Study the drawing (mm; zero at the part's minimum x, y, z) and answer. A direction names the side the tool comes from. Coordinates: 2 decimals unless noted, no trailing zeros. Order: outer loops, then holes, each group sorted by start corner. A loop starts at its lowest first (then second) coordinate and runs counter-clockwise, first axis right, second up. Notation, with made-up numbers: M 62,76 L 107,76 A17 ccw 107,81 Z; hole C -15,64.5 d2. An arc over 180 degrees is marked long. Put each result on its own line as item: value.
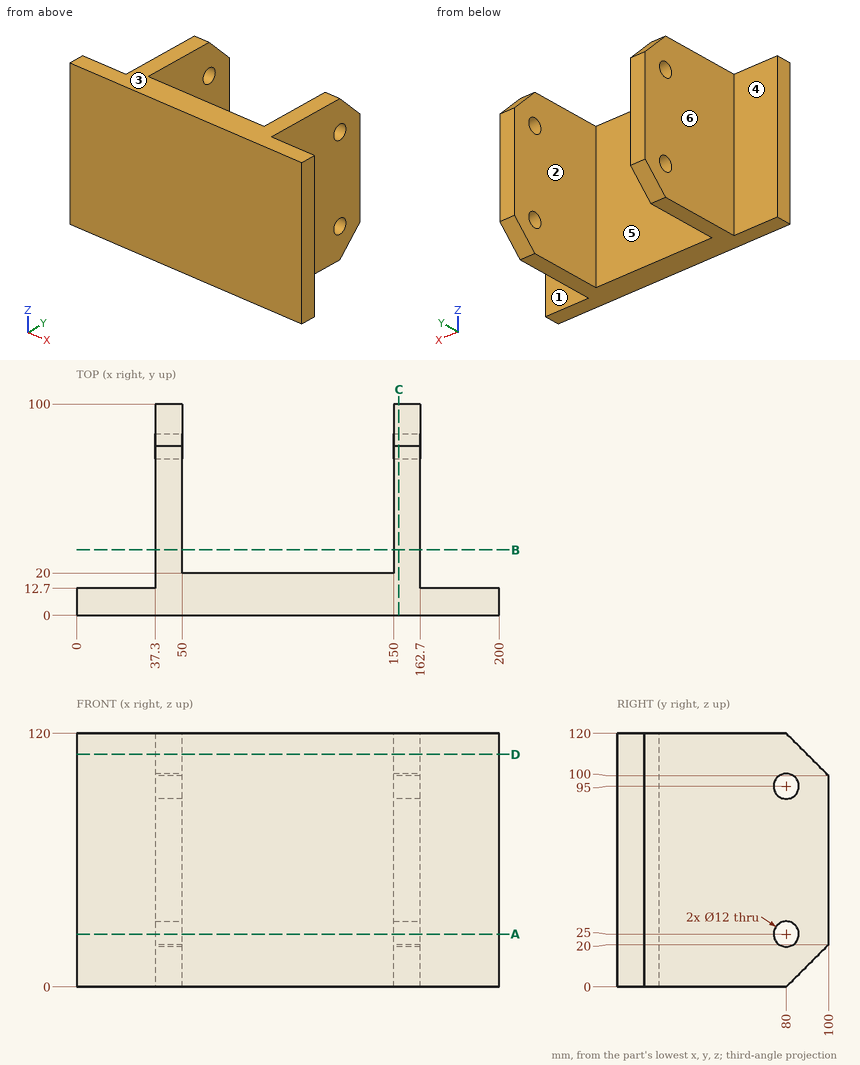
Q1. Find section A-A on z = 25. Write down the section's boundary in (x, y).
Answers below:
outline: M 0,0 L 200,0 L 200,12.7 L 162.7,12.7 L 162.7,74 L 150,74 L 150,20 L 50,20 L 50,74 L 37.3,74 L 37.3,12.7 L 0,12.7 Z; M 37.3,86 L 50,86 L 50,100 L 37.3,100 Z; M 150,86 L 162.7,86 L 162.7,100 L 150,100 Z
Q2. A tool of negligible diameter and unlimited length cuts with its end or side. For the marked faces 1, 2 and 3, from which of +Z, -Z, +X, -X, +Y, -Y can it reach the whole face along a straight path? Write none if from no direction.
Answers below:
face 1: +Z, -Z, +X, +Y
face 2: +Z, -Z, +Y
face 3: +Z, +X, -X, +Y, -Y
Q3. Find section D-D on z = 110. Write down the section's boundary in (x, y).
Answers below:
outline: M 0,0 L 200,0 L 200,12.7 L 162.7,12.7 L 162.7,90 L 150,90 L 150,20 L 50,20 L 50,90 L 37.3,90 L 37.3,12.7 L 0,12.7 Z
Q4. Find section B-B on y = 31. Write down the section's boundary in (x, z), plus the area to 3 significant figures.
Answers below:
outline: M 37.3,0 L 50,0 L 50,120 L 37.3,120 Z; M 150,0 L 162.7,0 L 162.7,120 L 150,120 Z
area: 3,050 mm^2
Q5. Consider line 1 along X through (y, z) = (57.5, 86.5); line 2 along Y through (x, z) = (156, 95); line 3 along Y through (x, z) = (136, 99.5). Determine where each line is inside the solid, lowest interval first.
Answers below:
line 1: x = 37.3 to 50, 150 to 162.7
line 2: y = 0 to 74, 86 to 100
line 3: y = 0 to 20
Q6. Find section C-C on x = 152.5. Write down the section's boundary in (y, z).
Answers below:
outline: M 0,0 L 80,0 L 100,20 L 100,100 L 80,120 L 0,120 Z; hole C 80,25 d12; hole C 80,95 d12
Q7. For a pull along X with two mould halves and no side action, classify the marked faces 4, 5 and 6 as +X half, -X half, draft (parallel to the pull), parting line (faces both ways), or undercut.
Answers below:
face 4: draft
face 5: undercut
face 6: -X half
Q8. Given pin 1 (18.5 mm diameter, centred on x = 185.5, z = 45.5, fed in from +Y); pin 2 (14 mm diameter, centred on y = 80, z = 95, fed in from -X); pin 3 (8 mm diameter, centred on x = 80.5, z = 55, fed in from +Y), each flat-ended and moving along its own axis, determine where each tip first touches the part or whether it passes through.
Answers below:
pin 1: stops at y = 12.7
pin 2: stops at x = 37.3
pin 3: stops at y = 20
